```python
from build123d import *

# Parameters (mm, degrees)
SKETCH_1_W          = 50
SKETCH_1_H          = 40
EXTRUDE_1_DEPTH     = 8
SKETCH_2_R          = 1.65
CUT_EXTRUDE_1_DEPTH = 15
CUT_EXTRUDE_2_DEPTH = 1
SKETCH_5_R          = 2.5
CUT_EXTRUDE_3_DEPTH = 10


with BuildPart() as part:
    # Эскиз1 → Бобышка-Вытянуть1 (new body)
    with BuildSketch(Plane.XY):
        Rectangle(SKETCH_1_W, SKETCH_1_H)
    extrude(amount=EXTRUDE_1_DEPTH)

    # Эскиз2 → Вырез-Вытянуть1 (cut)
    with BuildSketch(Plane(origin=(25, 0, 0), x_dir=(0, 0, -1), z_dir=(1, 0, 0))):
        with Locations(Location((-4, 10, 0), (0, 0, 90))):
            Circle(SKETCH_2_R)
        with Locations(Location((-4, -10, 0), (0, 0, 90))):
            Circle(SKETCH_2_R)
    extrude(amount=-CUT_EXTRUDE_1_DEPTH, mode=Mode.SUBTRACT)

    # Эскиз4 → Вырез-Вытянуть2 (cut)
    with BuildSketch(Plane.XY.offset(8)):
        with BuildLine():
            Line((-10, 20), (10, 20))
            Line((10, 20), (10, 10))
            ThreePointArc((10, 10), (0, 0), (-10, 10))
            Line((-10, 10), (-10, 20))
        make_face()
    extrude(amount=-CUT_EXTRUDE_2_DEPTH, mode=Mode.SUBTRACT)

    # Эскиз5 → Вырез-Вытянуть3 (cut)
    with BuildSketch(Plane.XY.offset(7)):
        with Locations((0, 16)):
            Circle(SKETCH_5_R)
    extrude(amount=-CUT_EXTRUDE_3_DEPTH, mode=Mode.SUBTRACT)


solid = part.part
```
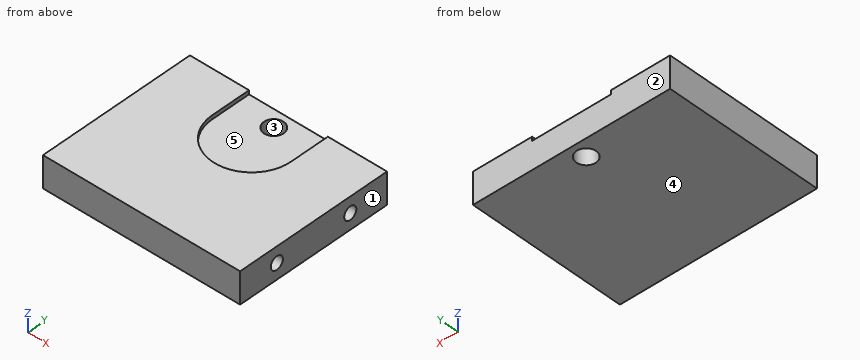
Source: CAD feature listing. Evaluate the final solid. Frame: model axes, mm. Face numbers are marked on the shaded views. A direction names the side the tool comes from. Coordinates: 2 decimals unless noted, no trailing zeros. Write each loop counter-clockwise with the first axis right and the second up, starting at its lowest first coordinate (ties: lowest second). Pieces come first, ordered by that corner, then holes. Notation, with made-up numbers: M 53.25,64 L 65.25,64 A23 ccw 65.25,97 Z; hole C -14.5,-29.5 d5. An arc over 180 degrees is marked long. Answer as a JSON object with one key per item and string values.
1. Cut plane A-A on x = 22. Output: boundary loops of the cut face in (y, z), plus the area to 3 significant figures.
Evaluation:
{"outline": "M -20,0 L 20,0 L 20,8 L -20,8 Z; hole C -10,4 d3.3; hole C 10,4 d3.3", "area": "303 mm^2"}
2. Cut plane D-D on y = -10. Output: boundary loops of the cut face in (x, z).
Evaluation:
{"outline": "M -25,0 L 25,0 L 25,2.35 L 10,2.35 L 10,5.65 L 25,5.65 L 25,8 L -25,8 Z"}
3. Access query for the marked faces 4 and 5. Directions: +Z, -Z, +X, -X, +Y, -Y. A direction counts if a zero-diameter tool reaches every point of the face in a straight line with its end or side. Return the directions, or none.
Evaluation:
{"face 4": "-Z, +X, -X, +Y, -Y", "face 5": "+Z, +Y"}
4. Contact query for a flat-ended pin moving along its axis: P1, Ø1.6, axis at y = 10, z = 3.5, coming from the +X side. Output: stop coordinate, or through.
Evaluation:
{"P1": "x = 10"}
5. Cut plane B-B on z = 4. Output: boundary loops of the cut face in (x, y), plus the area to 3 significant figures.
Evaluation:
{"outline": "M -25,-20 L 25,-20 L 25,-11.65 L 10,-11.65 L 10,-8.35 L 25,-8.35 L 25,8.35 L 10,8.35 L 10,11.65 L 25,11.65 L 25,20 L -25,20 Z; hole C 0,16 d5", "area": "1,880 mm^2"}
6. Ray query, L1, parallel to Z at x = 15, y = -10; L2, parallel to X at y = 17.5, z = 7.5; L3, parallel to X at y = 17, z = 5.75. Return the intervals inside material, ascending.
Evaluation:
{"L1": "0 to 2.35, 5.65 to 8", "L2": "-25 to -10, 10 to 25", "L3": "-25 to -2.29, 2.29 to 25"}
7. Draft query along Y for the marked faces 1, 2 and 3. Return one class per face: released by +Y, released by -Y, zero draft, split by the parting line, or undercut.
Evaluation:
{"face 1": "zero draft", "face 2": "released by +Y", "face 3": "undercut"}
8. Cut plane C-C on y = 16. Output: boundary loops of the cut face in (x, z).
Evaluation:
{"outline": "M -25,0 L -2.5,0 L -2.5,7 L -10,7 L -10,8 L -25,8 Z; M 2.5,0 L 25,0 L 25,8 L 10,8 L 10,7 L 2.5,7 Z"}
